Study the drawing (mm; zero at the part's minimum x, y, z) and answer. Round coordinates to 2 decimals unless told otherwise and drop trailing zeros. Write each loop counter-clockwise with the first axis right and the second up, starting at its lowest first coordinate (ties: lowest second). Pieces come first, ordered by that corner, then holes.
(1) A cutting plane is placed at B-B, the plane z = 11.75. Give the vertices of the cut face in (x, y).
(2) A cutting plane is placed at A-A, the plane x = 5.5. Give the vertices of the cut face in (y, z), and give its area (3 significant figures).
(3) This flat-tipped pin is pushed along its axis until it touches: pin 1 Ø6 at (x, y) = (29.5, 36) entering from -Z. Where does it stop, or does it pass through?
(4) Find the intervals of material crossed by probe 1 along Y at (x, z) = (7.5, 14), in increasing order.
(5) The mould has two halves that part along Z. Classify the marked faces 1, 2 and 3: +Z half, -Z half, draft (parallel to the pull), parting line (faces both ways), or undercut.
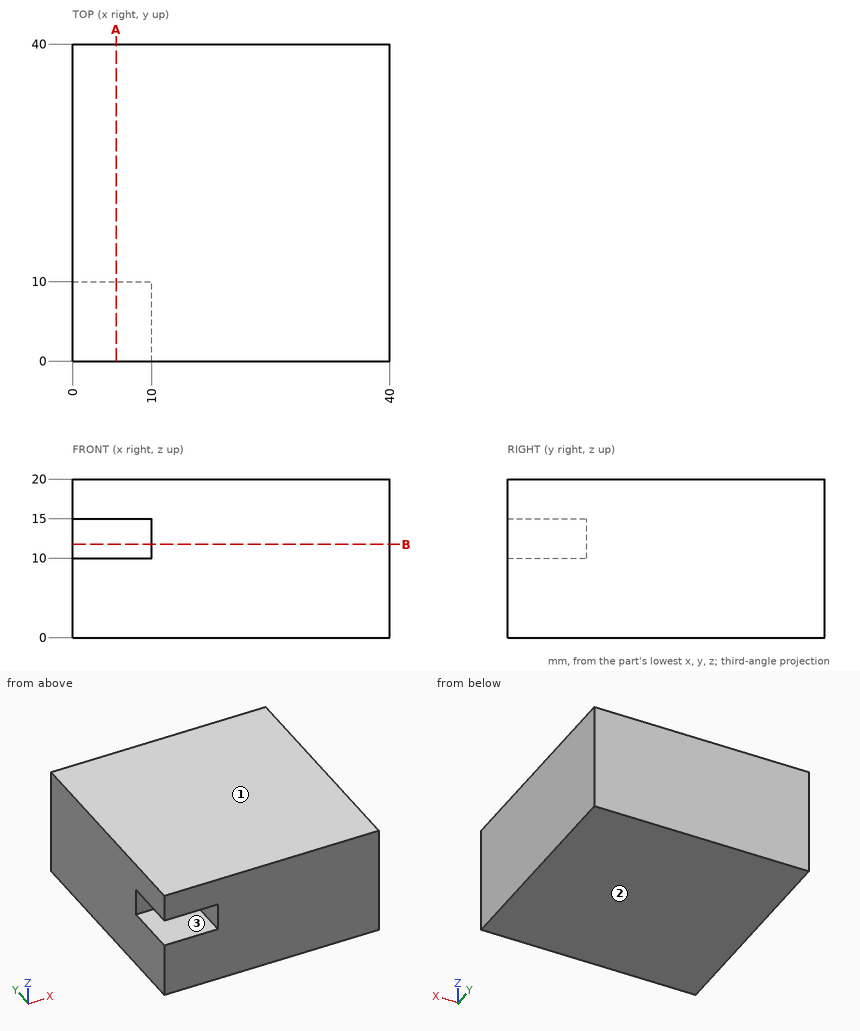
Solutions:
1. outline: (0, 10) - (10, 10) - (10, 0) - (40, 0) - (40, 40) - (0, 40) - close
2. outline: (0, 0) - (40, 0) - (40, 20) - (0, 20) - (0, 15) - (10, 15) - (10, 10) - (0, 10) - close
2. area: 750 mm2
3. pin 1: stops at z = 0
4. probe 1: y = 10 to 40
5. face 1: +Z half
5. face 2: -Z half
5. face 3: undercut
